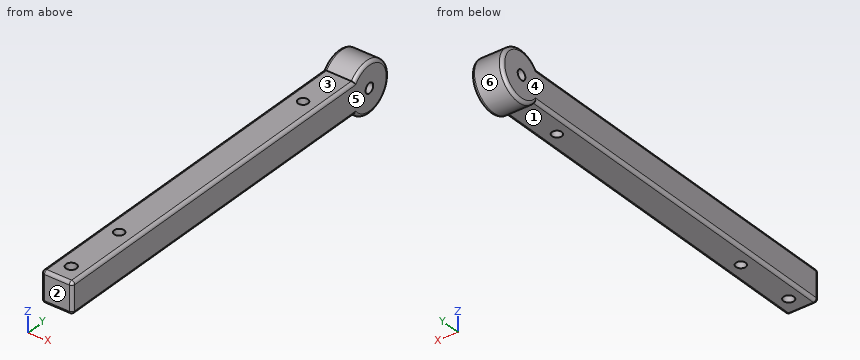
from build123d import *

# Parameters (mm, degrees)
SKETCH2_W           = 12.7
SKETCH2_H           = 165.1
BOSS_EXTRUDE1_DEPTH = 12.7
SKETCH4_R           = 10.16
BOSS_EXTRUDE2_DEPTH = 12.7
SKETCH5_R           = 2.032
CUT_EXTRUDE2_DEPTH  = 95.410065275
SKETCH6_R           = 2.159
CUT_EXTRUDE4_DEPTH  = 131.374531448
FILLET1_R           = 1.27
SKETCH7_R           = 2.032
CUT_EXTRUDE5_DEPTH  = 131.37453153


with BuildPart() as part:
    # Sketch2 → Boss-Extrude1 (new body)
    with BuildSketch(Plane.XY):
        with Locations((-84.455, -9.533605084)):
            Rectangle(SKETCH2_W, SKETCH2_H)
    extrude(amount=BOSS_EXTRUDE1_DEPTH)

    # Sketch4 → Boss-Extrude2 (add)
    with BuildSketch(Plane.ZY.offset(90.805)):
        with Locations((6.35, 65.396394916)):
            Circle(SKETCH4_R)
    extrude(amount=-BOSS_EXTRUDE2_DEPTH)

    # Sketch5 → Cut-Extrude2 (cut, through all)
    with BuildSketch(Plane.ZY.offset(90.805)):
        with Locations((6.35, 65.396394916)):
            Circle(SKETCH5_R)
    extrude(amount=-CUT_EXTRUDE2_DEPTH, mode=Mode.SUBTRACT)

    # Sketch6 → Cut-Extrude4 (cut, through all)
    with BuildSketch(Plane.XY.offset(12.7)):
        with Locations((-84.455, -84.463605084)):
            Circle(SKETCH6_R)
        with Locations((84.455, -84.463605084)):
            Circle(SKETCH6_R)
    extrude(amount=-CUT_EXTRUDE4_DEPTH, mode=Mode.SUBTRACT)

    # Fillet1
    fillet1_edges = [part.edges().sort_by_distance(p)[0] for p in [
        (-90.805, -17.309178813, 0),
        (-90.805, -17.309178813, 12.7),
        (-90.805, 75.556394916, 6.35),
        (-78.105, 75.556394916, 6.35),
        (-84.455, -92.083605084, 12.7),
        (-78.105, -17.309178813, 0),
        (-84.455, -92.083605084, 0),
        (-90.805, -92.083605084, 6.35),
        (-78.105, -92.083605084, 6.35),
        (-78.105, -17.309178813, 12.7),
    ]]
    fillet(fillet1_edges, radius=FILLET1_R)

    # Sketch7 → Cut-Extrude5 (cut, through all)
    with BuildSketch(Plane.XY.offset(12.7)):
        with Locations((-84.455, -59.063605084)):
            Circle(SKETCH7_R)
        with Locations((-84.455, 38.415247458)):
            Circle(SKETCH7_R)
        with Locations((84.455, -59.063605084)):
            Circle(SKETCH7_R)
        with Locations((84.455, 38.415247458)):
            Circle(SKETCH7_R)
    extrude(amount=-CUT_EXTRUDE5_DEPTH, mode=Mode.SUBTRACT)


solid = part.part
Input: part model. Units: mm. Frame: model coordinates. Face numbers are marked on the shaded views. A direction names the side the tool comes from. Round coordinates to 2 decimals unless told otherwise and drop trailing zeros. Order: outer loops, then holes, each group sorted by start corner. A loop starts at its lowest first (then second) coordinate and runs counter-clockwise, first axis right, second up. Notation, with made-up numbers: (25.5, 42.25) - (29.5, 42.25) arc R29 ccw to (29.5, 63.25) - close; hole circle Ø11 at (79.25, 80). An arc over 180 degrees is marked (long way). Answer as a JSON object with one key per item and string values. Group by question number.
(1) Cut plane B-B (z = 6.35). Return loops of the section in (x, y) (3 decimals).
(2) Cut plane A-A (y = -52). Return loops of the section in (x, z) (3 decimals).
(3) Reachability of the marked faces 1, 2 and 3 from +Z, -Z, +X, -X, +Y, -Y: full face, straight path, thin tool, end or side. Return the list, or none.
(4) Draft query along X for the marked faces 4, 5 and 6. Return one class per face: released by +X, released by -X, zero draft, split by the parting line, or undercut.
(5) Material intervals for probe 1 along Y at (x, z) = (-84.5, 6.5); probe 2 along Y at (x, z) = (-81.5, 6.35); probe 3 along Y at (x, z) = (-83.25, 5), sorted ascending. Write a range as from..to.
(6) Pin query (flat end, axial travel): P1, Ø4.5, axis at x = -84.46, y = 38.42, coming from the +Z side; P2, Ø6, axis at x = -85, y = 50.5, coming from the -Z side; P3, Ø3.5, axis at x = -84.46, y = -59.06, coming from the +Z side; P4, Ø1, axis at y = -47, z = 12, coming from the +X side. Return the tip coordinate at first contact, or that it passes through.
Here are the results:
{
 "1": {"outline": "(-90.805, -90.814) arc R1.27 ccw to (-89.535, -92.084) - (-79.375, -92.084) arc R1.27 ccw to (-78.105, -90.814) - (-78.105, 63.364) - (-90.805, 63.364) - close; (-90.805, 67.428) - (-78.105, 67.428) - (-78.105, 74.286) arc R1.27 ccw to (-79.375, 75.556) - (-89.535, 75.556) arc R1.27 ccw to (-90.805, 74.286) - close; hole circle Ø4.318 at (-84.455, -84.464); hole circle Ø4.064 at (-84.455, -59.064); hole circle Ø4.064 at (-84.455, 38.415)"},
 "2": {"outline": "(-90.805, 1.27) arc R1.27 ccw to (-89.535, 0) - (-79.375, 0) arc R1.27 ccw to (-78.105, 1.27) - (-78.105, 11.43) arc R1.27 ccw to (-79.375, 12.7) - (-89.535, 12.7) arc R1.27 ccw to (-90.805, 11.43) - close"},
 "3": {"face 1": "-Z, +X, -X, -Y", "face 2": "+Z, -Z, +X, -X, -Y", "face 3": "+Z, +X, -X, -Y"},
 "4": {"face 4": "released by -X", "face 5": "released by +X", "face 6": "zero draft"},
 "5": {"probe 1": "y = -92.08..-86.62, -82.31..-61.1, -57.03..36.38, 40.45..63.37, 67.42..75.56", "probe 2": "y = -92.08..63.36, 67.43..75.56", "probe 3": "y = -92.08..-86.26, -82.67..-60.7, -57.43..36.78, 40.05..63.88, 66.92..75.47"},
 "6": {"P1": "stops at z = 12.7", "P2": "stops at z = 0", "P3": "passes through", "P4": "stops at x = -78.11"}
}
